Input: dimensioned drawing with shaded views. Units: mm. Origin: part minimum x, y, z. A direction names the side the tool comes from. Round coordinates to 2 decimals unless told otherwise and drop trailing zeros. Write each loop counter-clockwise with the first axis right and the second up, starting at its lowest first coordinate (ties: lowest second). Pieces come first, ordered by that corner, then holes. Notation, with made-up numbers: (44.5, 45) - (82.5, 45) arc R21 cw to (82.5, 63) - close; hole circle Ø9 at (-17.5, -9.75). An arc over 180 degrees is marked (long way). Use one line per item in the form item = value.
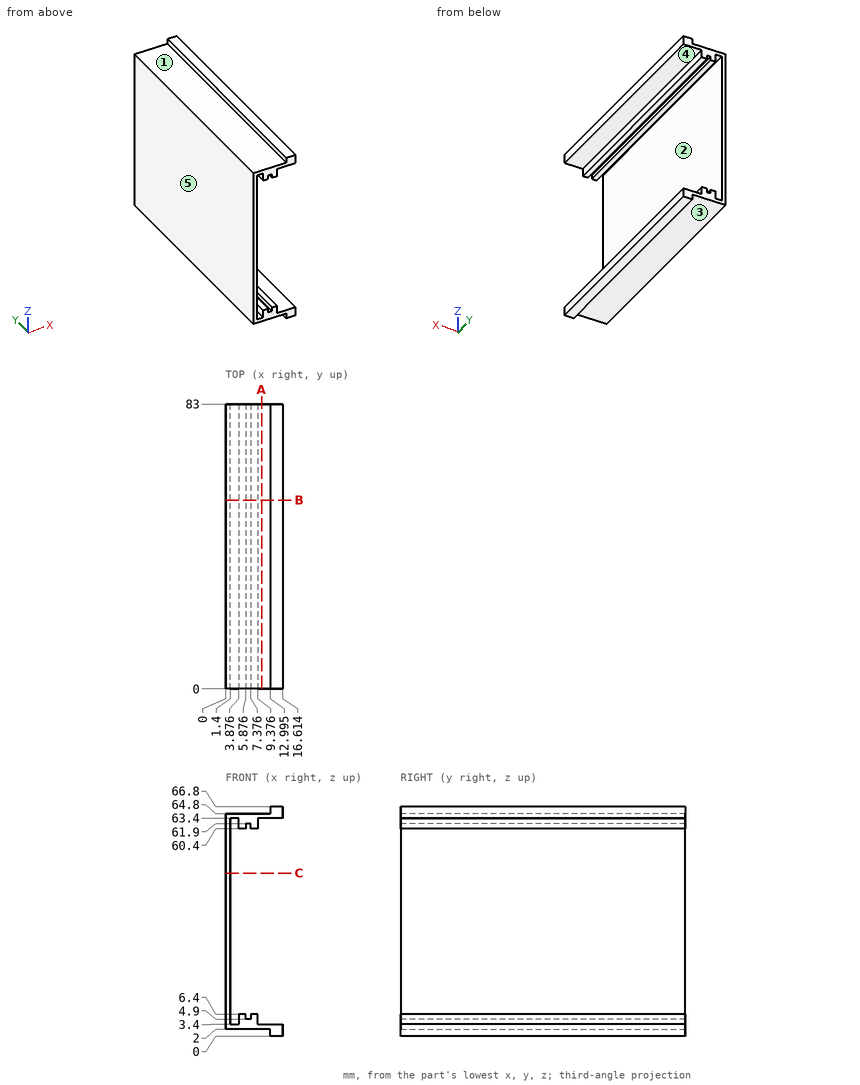
(1) Cut plane A-A on x = 10.5. Output: boundary loops of the cut face in (y, z).
Derived:
outline = (0, 2) - (83, 2) - (83, 3.4) - (0, 3.4) - close; (0, 63.4) - (83, 63.4) - (83, 64.8) - (0, 64.8) - close
(2) Access query for the marked faces 4 and 5. Directions: +Z, -Z, +X, -X, +Y, -Y. A direction counts if a zero-diameter tool reaches every point of the face in a straight line with its end or side. Return the directions, or none.
Derived:
face_4 = +X, +Y, -Y
face_5 = +Z, -Z, -X, +Y, -Y
(3) Cut plane C-C on z = 47.5. Output: boundary loops of the cut face in (x, y), then the cut area to 3 significant figures.
Derived:
outline = (0, 0) - (1.4, 0) - (1.4, 83) - (0, 83) - close
area = 116 mm^2
(4) Draft query along Z for the marked faces 1, 2 and 3. Return one class per face: released by +Z, released by -Z, zero draft, split by the parting line, or undercut.
Derived:
face_1 = released by +Z
face_2 = undercut
face_3 = released by -Z
(5) First-contact query: pin 1 Ø8 at (x, y) = (7.5, 41.5) entering from -Z; pin 2 Ø1.6 at (y, z) = (27.5, 5.5) entering from +X; pin 3 Ø1.6 at (x, y) = (8.5, 53) entering from +Z. Flat tips, straight axial feed; report the tip coordinate or a pass-through.
Derived:
pin_1 = 2
pin_2 = 9.38
pin_3 = 64.8
(6) Material intervals for L1, parallel to Z at x = 3.75, y = 50.5; L2, parallel to X at y = 31, z = 62; L3, parallel to Z at x = 4.5, y = 50, sorted ascending.
Derived:
L1 = 2 to 3.4, 63.4 to 64.8
L2 = 0 to 1.4, 3.88 to 9.38
L3 = 2 to 6.4, 60.4 to 64.8
(7) Cut plane B-B on y = 55. Output: boundary loops of the cut face in (x, z) (3 decimals).
Derived:
outline = (0, 2) - (12.995, 2) - (12.995, 0) - (16.614, 0) - (16.614, 3.4) - (9.376, 3.4) - (9.376, 6.4) - (7.376, 6.4) - (7.376, 4.9) - (5.876, 4.9) - (5.876, 6.4) - (3.876, 6.4) - (3.876, 3.4) - (1.4, 3.4) - (1.4, 63.4) - (3.876, 63.4) - (3.876, 60.4) - (5.876, 60.4) - (5.876, 61.9) - (7.376, 61.9) - (7.376, 60.4) - (9.376, 60.4) - (9.376, 63.4) - (16.614, 63.4) - (16.614, 66.8) - (12.995, 66.8) - (12.995, 64.8) - (0, 64.8) - close
